Can you work these out from the model? Positions are in its coordinate system, mm. A direction names the side the tool comes from. Coordinates: 2 decimals unless noted, no trailing zeros. Order: outer loops, then holes, each group sorted by start corner. A loop starts at its lowest first (then second) coordinate and runs counter-clockwise, first axis right, second up.
```python
from build123d import *

# Parameters (mm, degrees)
F0_R     = 26.035
F0_R_2   = 24.13
F1_DEPTH = 1.27
F2_R     = 0.254
F3_DEPTH = 12.7


with BuildPart() as f1:
    # F0 (on Front) → F1 (new body, symmetric)
    with BuildSketch(Plane.XZ):
        Circle(F0_R)
        Circle(F0_R_2, mode=Mode.SUBTRACT)
    extrude(amount=F1_DEPTH, both=True)

    # F2 (on Front) → F3 (cut, symmetric)
    with BuildSketch(Plane.XZ):
        with BuildLine():
            Line((-24.1269919178, 0.381), (-26.0322120458, 0.381))
            ThreePointArc((-26.0322120458, 0.381), (-26.035, 0), (-26.0322120458, -0.381))
            Line((-26.0322120458, -0.381), (-24.1269919178, -0.381))
            ThreePointArc((-24.1269919178, -0.381), (-24.13, 0), (-24.1269919178, 0.381))
        make_face()
        with Locations((-25.0796019818, -1.016)):
            Circle(F2_R)
        with Locations((-25.0796019818, 1.016)):
            Circle(F2_R)
    extrude(amount=F3_DEPTH, both=True, mode=Mode.SUBTRACT)


solid = f1.part
```
1. I'm going to push flat-ended pins straight in: pin 1 (1 mm diameter, centred on x = 16.5, y = 0.5, fed in from -Z); pin 2 (1.5 mm diameter, centred on x = -24.5, y = 0, fed in from +Z). Where does each tip first touch, or does it pass through?
Completed:
pin 1: stops at z = -20.54
pin 2: stops at z = 10.67
2. Imagine slicing it at A-A on x = 0. Please give me the cut outline in (y, z) (3 decimals), then the cut area to 3 significant figures.
Completed:
outline: (-1.27, -26.035) - (1.27, -26.035) - (1.27, -24.13) - (-1.27, -24.13) - close; (-1.27, 24.13) - (1.27, 24.13) - (1.27, 26.035) - (-1.27, 26.035) - close
area: 9.68 mm2
3. Please list where these lines run through material, in increasing order: probe 1 along Z at (x, y) = (12, -0.85); probe 2 along Z at (x, y) = (-22, -0.8).
Completed:
probe 1: z = -23.1 to -20.93, 20.93 to 23.1
probe 2: z = -13.92 to -9.91, 9.91 to 13.92
4. Imagine slicing it at C-C on y = 0.6. Please give me the cut outline in (x, z) (3 decimals).
Completed:
outline: (-26.032, -0.381) arc R26.035 ccw (long way) to (-26.032, 0.381) - (-24.127, 0.381) arc R24.13 cw (long way) to (-24.127, -0.381) - close; hole circle Ø0.508 at (-25.08, -1.016); hole circle Ø0.508 at (-25.08, 1.016)
5. On a 3-axis mill with a long thin cutter (end or side, diameter ignored), from which of +Z, -Z, +X, -X, +Y, -Y can I reach the whole of each face in a straight line? I mean faces 1 (the flat face through (-25, 0, -0.381)), 2 (the flat face through (23, 1.27, -8)). Say none if no direction works.
Completed:
face 1: -X, +Y, -Y
face 2: +Z, -Z, +X, -X, +Y
6. Imagine slicing it at B-B on z = -14. Please give me the cut outline in (x, y).
Completed:
outline: (-21.95, -1.27) - (-19.65, -1.27) - (-19.65, 1.27) - (-21.95, 1.27) - close; (19.65, -1.27) - (21.95, -1.27) - (21.95, 1.27) - (19.65, 1.27) - close
7. Thinking about a two-plate mould opening in Z: for faces 3 (the flat face through (-25, 0, 0.381)), 4 (the flat face through (23, -1.27, -8)), which applies, pulls with the +Z half, pulls with the -Z half, needs draft (parallel to the pull), parting line crosses it, or undercut?
Completed:
face 3: undercut
face 4: needs draft
